from build123d import *

# Parameters (mm, degrees)
F0_W     = 60
F0_H     = 40
F3_DEPTH = 10
F1_W     = 20
F1_H     = 40
F4_DEPTH = 30
F2_W     = 20
F2_H     = 10
F5_DEPTH = 20


with BuildPart() as f3:
    # F0 (on Top) → F3 (new body)
    with BuildSketch(Plane.XY):
        with Locations((30, 20)):
            Rectangle(F0_W, F0_H)
    extrude(amount=F3_DEPTH)

    # F1 (on Top) → F4 (join)
    with BuildSketch(Plane.XY):
        with Locations((10, 20)):
            Rectangle(F1_W, F1_H)
    extrude(amount=F4_DEPTH)

    # F2 (on Top) → F5 (join)
    with BuildSketch(Plane.XY):
        with Locations((29.928178, 5)):
            Rectangle(F2_W, F2_H)
        with Locations((30.014171, 35)):
            Rectangle(F2_W, F2_H)
    extrude(amount=F5_DEPTH)


solid = f3.part
Could you check a few things on this model? Use its own coordinates, in mm. A direction names the side the tool comes from. Give positions to 0.01 mm unless a question says otherwise; leave off trailing zeros. Loops run counter-clockwise (first coordinate to the right, second up) from the corner with the lowest first, then second, coordinate; pieces in that order, holes last. Notation, with made-up numbers: M -39.5,26.5 L -26.5,26.5 A12 ccw -26.5,48.5 Z; hole C -27,11.5 d9. An arc over 180 degrees is marked long. Answer as a JSON object with one key per item and string values.
Q1. Suppose I cut it at A-A, the plane z = 17.5. List the corners of the cut face in (x, y) for me, plus the area to 3 significant figures.
Values found:
{"outline": "M 0,0 L 39.93,0 L 39.93,10 L 20,10 L 20,40 L 0,40 Z; M 20.01,30 L 40.01,30 L 40.01,40 L 20.01,40 Z", "area": "1,200 mm²"}
Q2. For faces 5 (the flat face through (10, 20, 30)), 6 (the flat face through (30, 30, 15)), 7 (the flat face through (30, 35, 20)), 8 (the flat face through (39.928, 5, 15)), which set-ups out of +Z, -Z, +X, -X, +Y, -Y let a thin tool reach every point of the face, with its end or its side?
Values found:
{"face 5": "+Z, +X, -X, +Y, -Y", "face 6": "+Z, +X", "face 7": "+Z, +X, +Y, -Y", "face 8": "+Z, +X, -Y"}
Q3. Suppose I cut it at B-B, the plane x = 36. List the corners of the cut face in (y, z) for me.
Values found:
{"outline": "M 0,0 L 40,0 L 40,20 L 30,20 L 30,10 L 10,10 L 10,20 L 0,20 Z"}
Q4. Suppose I cut it at D-D, the plane z = 22.5. List the corners of the cut face in (x, y) for me.
Values found:
{"outline": "M 0,0 L 20,0 L 20,40 L 0,40 Z"}
Q5. If we mould it in two halves opening along Y, with no side actions, what happens to faces 1 (the flat face through (23, 40, 11)), 2 (the flat face through (44, 20, 10)), 3 (the flat face through (30, 5, 20)), 4 (the flat face through (30, 10, 15))? For each: pulls with the +Y half, pulls with the -Y half, needs draft (parallel to the pull), parting line crosses it, or undercut.
Values found:
{"face 1": "pulls with the +Y half", "face 2": "undercut", "face 3": "needs draft", "face 4": "undercut"}
Q6. If I drill on probe 1 along Z at (x, y) = (55.5, 16.5); probe 2 along X at (y, z) = (8, 10.5); probe 3 along X at (y, z) = (13.5, 15.25), over which ranges is the centre line in solid material (lowest first)? Write a range as [from, to].
Values found:
{"probe 1": "z = [0, 10]", "probe 2": "x = [0, 39.93]", "probe 3": "x = [0, 20]"}
Q7. For P1, Ø5, axis at y = 5.5, z = 15, coming from the +X side; P2, Ø11, axis at x = 34.5, y = 37.5, coming from the +Z side; P3, Ø3, axis at y = 34.5, z = 14, coming from the +X side, each with a flat end and sliding along its axis, tell me the tip position at first contact or that it passes through.
Values found:
{"P1": "stops at x = 39.93", "P2": "stops at z = 20", "P3": "stops at x = 40.01"}
